```python
from build123d import *

# Parameters (mm, degrees)
BOSS_EXTRUDE1_DEPTH = 16.1
CUT_EXTRUDE1_DEPTH  = 32.2
SKETCH3_R           = 3.935
SKETCH3_R_2         = 1
CUT_EXTRUDE2_DEPTH  = 32.2
SKETCH4_R           = 3.935
SKETCH4_R_2         = 1
CUT_EXTRUDE3_DEPTH  = 32.2
CHAMFER1_SIZE       = 6
CHAMFER2_SIZE       = 7


with BuildPart() as part:
    # Sketch1 → Boss-Extrude1 (new, symmetric)
    with BuildSketch(Plane(origin=(0, 0, 0), x_dir=(1, 0, 0), z_dir=(0, 1, 0))):
        Polygon((0, 0), (-21.25, 0), (-21.25, -52.5), (-19.03, -52.5), (-19.03, -2.22), (0, -2.22), align=None)
    boss_extrude1 = extrude(amount=BOSS_EXTRUDE1_DEPTH, both=True)

    # Sketch2 → Cut-Extrude1 (cut)
    with BuildSketch(Plane.ZY.offset(21.25)):
        Polygon((43.03, 16.1), (52.5, 6.63), (52.5, 16.1), align=None)
        Polygon((52.5, -6.63), (43.03, -16.1), (52.5, -16.1), align=None)
    cut_extrude1 = extrude(amount=-CUT_EXTRUDE1_DEPTH, mode=Mode.SUBTRACT)

    # Sketch3 → Cut-Extrude2 (cut)
    with BuildSketch(Plane.ZY.offset(21.25)):
        with Locations((39.5, 0)):
            Circle(SKETCH3_R)
        with Locations((34.5, 5)):
            Circle(SKETCH3_R_2)
        with Locations((44.5, 5)):
            Circle(SKETCH3_R_2)
        with Locations((44.5, -5)):
            Circle(SKETCH3_R_2)
        with Locations((34.5, -5)):
            Circle(SKETCH3_R_2)
    cut_extrude2 = extrude(amount=-CUT_EXTRUDE2_DEPTH, mode=Mode.SUBTRACT)

    # Mirror1: Boss-Extrude1, Cut-Extrude1, Cut-Extrude2 across plane
    add(boss_extrude1.mirror(Plane(origin=(0, 16.1, 2.22), x_dir=(0, 0, 1), z_dir=(-1, 0, 0))))
    add(cut_extrude1.mirror(Plane(origin=(0, 16.1, 2.22), x_dir=(0, 0, 1), z_dir=(-1, 0, 0))), mode=Mode.SUBTRACT)
    add(cut_extrude2.mirror(Plane(origin=(0, 16.1, 2.22), x_dir=(0, 0, 1), z_dir=(-1, 0, 0))), mode=Mode.SUBTRACT)

    # Sketch4 → Cut-Extrude3 (cut)
    with BuildSketch(Plane.XY.offset(2.22)):
        Circle(SKETCH4_R)
        with Locations((-5, 5)):
            Circle(SKETCH4_R_2)
        with Locations((5, 5)):
            Circle(SKETCH4_R_2)
        with Locations((5, -5)):
            Circle(SKETCH4_R_2)
        with Locations((-5, -5)):
            Circle(SKETCH4_R_2)
        with Locations((-7.071067812, 0)):
            Circle(SKETCH4_R_2)
        with Locations((0, 7.071067812)):
            Circle(SKETCH4_R_2)
        with Locations((7.071067812, 0)):
            Circle(SKETCH4_R_2)
        with Locations((0, -7.071067812)):
            Circle(SKETCH4_R_2)
    extrude(amount=-CUT_EXTRUDE3_DEPTH, mode=Mode.SUBTRACT)

    # Chamfer1
    chamfer1_edges = [part.edges().sort_by_distance(p)[0] for p in [
        (-19.03, 0, 2.22),
        (19.03, 0, 2.22),
    ]]
    chamfer(chamfer1_edges, length=CHAMFER1_SIZE)

    # Chamfer2
    chamfer2_edges = [part.edges().sort_by_distance(p)[0] for p in [
        (-21.25, 0, 0),
        (21.25, 0, 0),
    ]]
    chamfer(chamfer2_edges, length=CHAMFER2_SIZE)


solid = part.part
```
Work out the finished part from the listing and answer in its coordinate system (mm). A direction names the side the tool comes from. Coordinates: 2 decimals unless noted, no trailing zeros. Loops run counter-clockwise (first coordinate to the right, second up) from the corner with the lowest first, then second, coordinate; pieces in that order, holes last.
1) For faces 4 (the flat face through (17.8, -0.23, 3.55)), 5 (the flat face through (-19.03, 0, 31)), determine the directions among +Z, -Z, +X, -X, +Y, -Y from which every point of the face is accessible in a straight line to the end or side of a thin tool.
Results:
face 4: -Z, +X, +Y, -Y
face 5: +Z, +Y, -Y
2) Section A-A (z = 30.5) is taken. Give the vertices of the cut face in (x, y).
Results:
outline: (-21.25, -16.1) - (-19.03, -16.1) - (-19.03, 16.1) - (-21.25, 16.1) - close; (19.03, -16.1) - (21.25, -16.1) - (21.25, 16.1) - (19.03, 16.1) - close
3) Section C-C (z = 39.5) is taken. Give the vertices of the cut face in (x, y) (3 decimals), plus the area to 3 significant figures.
Results:
outline: (-21.25, -16.1) - (-19.03, -16.1) - (-19.03, -3.935) - (-21.25, -3.935) - close; (-21.25, 3.935) - (-19.03, 3.935) - (-19.03, 16.1) - (-21.25, 16.1) - close; (19.03, -16.1) - (21.25, -16.1) - (21.25, -3.935) - (19.03, -3.935) - close; (19.03, 3.935) - (21.25, 3.935) - (21.25, 16.1) - (19.03, 16.1) - close
area: 108 mm2
4) Section B-B (x = -5) is taken. Give the vertices of the cut face in (y, z), plus the area to 3 significant figures.
Results:
outline: (-16.1, 0) - (-6, 0) - (-6, 2.22) - (-16.1, 2.22) - close; (-4, 0) - (4, 0) - (4, 2.22) - (-4, 2.22) - close; (6, 0) - (16.1, 0) - (16.1, 2.22) - (6, 2.22) - close
area: 62.6 mm2
5) Consider probe 1 along Y at (x, z) = (5, 0.75); probe 2 along Y at (x, z) = (0, 1.5) (3 decimals); probe 3 along X at (y, z) = (2, 44). Determine where each line is inside the solid, lowest interval first.
Results:
probe 1: y = -16.1 to -6, -4 to 4, 6 to 16.1
probe 2: y = -16.1 to -8.071, -6.071 to -3.935, 3.935 to 6.071, 8.071 to 16.1
probe 3: x = -21.25 to -19.03, 19.03 to 21.25
6) Flat-ended cylindrical pins translate along their axes: pin 1 (1.8 mm diameter, centred on x = -7.07, y = 0, fed in from -Z); pin 2 (1.5 mm diameter, centred on x = 15.5, y = -4.5, fed in from -Z); pin 3 (6 mm diameter, centred on x = -8.5, y = 4, fed in from +Z); pin 4 (12 mm diameter, centred on x = -8, y = -10, fed in from +Z). Find the tip coordinate at first contact, or state that the pin passes through.
Results:
pin 1: passes through
pin 2: stops at z = 0.5
pin 3: stops at z = 2.22
pin 4: stops at z = 3.19
7) For a pull along Z with two mould halves and no side action, classify faces 1 (the flat face through (-3, 4, 2.22)), 2 (the cylindrical face through (20.156, -1.507, 43.135)), 3 (the cylindrical face through (3.753, 1.182, 1.126)) as +Z half, -Z half, draft (parallel to the pull), parting line (faces both ways), or undercut.
Results:
face 1: +Z half
face 2: undercut
face 3: draft
8) Section D-D (y = 0) is taken. Give the number of separate pieces and of enclosed holes in the cut face, plus the area to 3 significant figures.
Results:
separate pieces: 6
enclosed holes: 0
area: 243 mm2
